from build123d import *

# Parameters (mm, degrees)
SKETCH1_R           = 2.85
BOSS_EXTRUDE1_DEPTH = 3
SKETCH2_R           = 1.5
BOSS_EXTRUDE2_DEPTH = 30
CHAMFER1_SIZE       = 0.3
CUT_EXTRUDE1_DEPTH  = 2


with BuildPart() as part:
    # Sketch1 → Boss-Extrude1 (new body)
    with BuildSketch(Plane.XY):
        Circle(SKETCH1_R)
    extrude(amount=BOSS_EXTRUDE1_DEPTH)

    # Sketch2 → Boss-Extrude2 (add)
    with BuildSketch(Plane(origin=(0, 0, 0), x_dir=(-1, 0, 0), z_dir=(0, 0, -1))):
        Circle(SKETCH2_R)
    extrude(amount=BOSS_EXTRUDE2_DEPTH)

    # Chamfer1
    chamfer1_edges = [part.edges().sort_by_distance(p)[0] for p in [
        (1.5, 0, -30),
    ]]
    chamfer(chamfer1_edges, length=CHAMFER1_SIZE)

    # Sketch3 → Cut-Extrude1 (cut)
    with BuildSketch(Plane.XY.offset(3)):
        Polygon((0, 1.443375673), (-1.25, 0.721687836), (-1.25, -0.721687836), (0, -1.443375673), (1.25, -0.721687836), (1.25, 0.721687836), align=None)
    extrude(amount=-CUT_EXTRUDE1_DEPTH, mode=Mode.SUBTRACT)


solid = part.part
Could you check a few things on this model? Use its own coordinates, in mm. A direction names the side the tool comes from. Give positions to 0.01 mm unless a question says otherwise; leave off trailing zeros. Order: outer loops, then holes, each group sorted by start corner. A loop starts at its lowest first (then second) coordinate and runs counter-clockwise, first axis right, second up. Notation, with made-up numbers: (7, -28) -> (49, -28) arc R6 cw to (49, -17) -> close; hole circle Ø4 at (19.5, 86). An arc over 180 degrees is marked (long way). Answer in a Markdown table with one row per item. Add a question column.
Item 1: Imagine slicing it at B-B (z = -9.5). List the corners of the cut face in (x, y) for me, and give its area (3 significant figures).
Item 2: For faces 5 (the flat face through (1.2, -1.2, 0)), 6 (the flat face through (1.25, 0, 2)), 7 (the flat face through (-0.67, -1.23, 3)), which set-ups out of +Z, -Z, +X, -X, +Y, -Y let a thin tool reach every point of the face, with its end or its side?
Item 3: I'm going to push a flat-ended pin straight in: P1, Ø0.8, axis at x = -0.5, y = -0.5, coming from the +Z side. Where does the tip first touch, or does it pass through?
Item 4: Please list where these lines run through material, in increasing order: probe 1 along Z at (x, y) = (2.2, 1.7); probe 2 along X at (y, z) = (0.9, -15.5); probe 3 along Z at (x, y) = (-0.65, -0.3).
Item 5: Imagine slicing it at A-A (y = 0). List the corners of the cut face in (x, z) for me, and give its area (3 significant figures).
Item 6: We'd pull the mould along Y, two halves only. Please class faces 1 (the flat face through (0.616, -1.088, 2.014)), 2 (the flat face through (0, 0, -30)), 3 (the cylindrical face through (-2.262, -1.734, 1.479)), 4 (the flat face through (-0.616, 1.088, 2.014)): pulls with the +Y half, pulls with the -Y half, needs draft (parallel to the pull), parting line crosses it, or undercut.
Result:
| question | item | result |
|---|---|---|
| 1 | outline | circle Ø3 at (0, 0) |
| 1 | area | 7.07 mm2 |
| 2 | face 5 | -Z |
| 2 | face 6 | +Z |
| 2 | face 7 | +Z, +X, -X, +Y, -Y |
| 3 | P1 | z = 1 |
| 4 | probe 1 | 0 to 3 |
| 4 | probe 2 | -1.2 to 1.2 |
| 4 | probe 3 | -30 to 1 |
| 5 | outline | (-2.85, 0) -> (-1.5, 0) -> (-1.5, -29.7) -> (-1.2, -30) -> (1.2, -30) -> (1.5, -29.7) -> (1.5, 0) -> (2.85, 0) -> (2.85, 3) -> (1.25, 3) -> (1.25, 1) -> (-1.25, 1) -> (-1.25, 3) -> (-2.85, 3) -> close |
| 5 | area | 102 mm2 |
| 6 | face 1 | undercut |
| 6 | face 2 | needs draft |
| 6 | face 3 | parting line crosses it |
| 6 | face 4 | undercut |
